Geometry check sheet. Reference: the model listing, model coordinates, mm. A direction names the side the tool comes from. Give positions to 0.01 mm unless a question says otherwise; leave off trailing zeros. Loops run counter-clockwise (first coordinate to the right, second up) from the corner with the lowest first, then second, coordinate; pieces in that order, holes last. Notation, with made-up numbers: (-22, -2.5) - (0, -2.5) arc R27 cw to (0, 35.5) - close; hole circle Ø7 at (83.25, 24). An arc over 180 degrees is marked (long way). Use a Markdown table: item, result. Add a question column.
1. Draft check along X on faces 6 (the cylindrical face through (6.3, 99.98, -32.47)), 7 (the flat face through (-1, 38, -32)), 8 (the flat face through (24.5, 14, -0.4)). Enter one of: pulls with the +X half, pulls with the -X half, needs draft (parallel to the pull), parting line crosses it, or undercut.
2. Cross-section at A-A on z = 0.5. Enter the section's corners in (x, y).
3. Material ranges on L1, parallel to Y at x = 16, z = -9; L2, parallel to Z at x = 11.5, y = 51; L3, parallel to X at y = 79, z = 2.5, recorded low to high.
4. Cross-section at C-C on z = 18. Enter the section's corners in (x, y).
5. Cross-section at B-B on y = 65.5. Enter the section's corners in (x, z).
6. Depth check by flat-ended pin: P1, Ø7.5, axis at x = 28.09, z = -0.34, coming from the +Y side; P2, Ø20, axis at x = 17.5, y = 41.5, coming from the +Z side; P3, Ø12, axis at x = 28.5, z = -1.5, coming from the +Y side. Enter the tip coordinate at first touch or a pass-through.
7. Set-up check for faces 1 (the cylindrical face through (-6.285, 99.993, -32.464)), 2 (the cylindrical face through (19.675, 87.022, -22.273)), 3 (the flat face through (-32, 75, -31)), 4 (the flat face through (32, 74, -31)), 5 (the cylindrical face through (22.726, 17.042, -1.534)): record each of +Z, -Z, +X, -X, +Y, -Y from which the full face is reachable in a straight line by a thin tool's end or side.
8. Cross-section at D-D on x = 41.5. Enter the section's corners in (y, z), and give its area (3 significant figures).
from build123d import *

# Parameters (mm, degrees)
SKETCH4_W                      = 96
SKETCH4_H                      = 64
BOSS_EXTRUDE1_DEPTH            = 20
BOSS_EXTRUDE2_DEPTH            = 32
BOSS_EXTRUDE3_DEPTH            = 12
SKETCH7_R                      = 26
SKETCH7_R_2                    = 16
BOSS_EXTRUDE4_DEPTH            = 32
CUT_EXTRUDE1_START             = -32
SKETCH8_R                      = 16
CUT_EXTRUDE1_DEPTH             = 32
RIB1_START                     = -6
RIB1_DEPTH                     = 12
FILLET1_R                      = 1
CBORE_FOR_M6_SHCS2_D           = 6.6
CBORE_FOR_M6_SHCS2_CBORE_D     = 11
CBORE_FOR_M6_SHCS2_CBORE_DEPTH = 6


with BuildPart() as part:
    # Sketch4 → Boss-Extrude1 (new body)
    with BuildSketch(Plane(origin=(0, 0, 0), x_dir=(1, 0, 0), z_dir=(0, 1, 0))):
        Rectangle(SKETCH4_W, SKETCH4_H)
    extrude(amount=BOSS_EXTRUDE1_DEPTH)

    # Sketch5 → Boss-Extrude2 (add, symmetric)
    with BuildSketch(Plane(origin=(0, 0, 0), x_dir=(0, 0, -1), z_dir=(1, 0, 0))):
        with BuildLine():
            Line((20, 0), (32, 0))
            Line((32, 0), (32, 76.178360588))
            ThreePointArc((32, 76.178360588), (33.228648741, 82.123937475), (36.713317934, 87.095510953))
            Line((36.713317934, 87.095510953), (63.616851895, 112.445358766))
            Line((63.616851895, 112.445358766), (55.387506243, 121.179079058))
            Line((55.387506243, 121.179079058), (28.483972282, 95.829231245))
            ThreePointArc((28.483972282, 95.829231245), (22.211567734, 86.880398983), (20, 76.178360588))
            Line((20, 76.178360588), (20, 0))
        make_face()
    extrude(amount=BOSS_EXTRUDE2_DEPTH, both=True)

    # Sketch6 → Boss-Extrude3 (add)
    with BuildSketch(Plane(origin=(0, 36.544630029, 34.434168053), x_dir=(1, 0, 0), z_dir=(0, 0.7278100243036815, 0.6857788043699474))):
        with BuildLine():
            Line((-32, 123.413626216), (32, 123.413626216))
            ThreePointArc((32, 123.413626216), (0, 155.413626216), (-32, 123.413626216))
        make_face()
    extrude(amount=-BOSS_EXTRUDE3_DEPTH)

    # Sketch7 → Boss-Extrude4 (add)
    with BuildSketch(Plane(origin=(0, 36.544630029, 34.434168053), x_dir=(1, 0, 0), z_dir=(0, 0.7278100243036815, 0.6857788043699474))):
        with Locations(Location((0, 123.413626216, 0), (0, 0, 270))):
            Circle(SKETCH7_R)
        with Locations(Location((0, 123.413626216, 0), (0, 0, 270))):
            Circle(SKETCH7_R_2, mode=Mode.SUBTRACT)
    extrude(amount=BOSS_EXTRUDE4_DEPTH)

    # Sketch8 → Cut-Extrude1 (cut)
    with BuildSketch(Plane(origin=(0, 36.544630029, 34.434168053), x_dir=(1, 0, 0), z_dir=(0, 0.7278100243036815, 0.6857788043699474)).offset(CUT_EXTRUDE1_START)):
        with Locations(Location((0, 123.413626216, 0), (0, 0, 270))):
            Circle(SKETCH8_R)
    extrude(amount=CUT_EXTRUDE1_DEPTH, mode=Mode.SUBTRACT)

    # Rib1: read off the stored shape, not the designer's step
    # Rib1 outline → Rib1 (add)
    with BuildSketch(Plane(origin=(0, 0, 0), x_dir=(0, 0, -1), z_dir=(1, 0, 0)).offset(RIB1_START)):
        with BuildLine():
            Line((28.483972282, 95.829231245), (36.975207197, 103.830095115))
            Line((36.975207197, 103.830095115), (19.144958284, 122.753155747))
            Line((19.144958284, 122.753155747), (10.653723368, 114.752291877))
            ThreePointArc((10.653723368, 114.752291877), (-1.658774448, 97.186065586), (-6, 76.178360588))
            ThreePointArc((-6, 76.178360588), (-12.815134364, 45.226752398), (-32, 20))
            Line((-32, 20), (20, 20))
            Line((20, 20), (20, 76.178360588))
            ThreePointArc((20, 76.178360588), (22.211567734, 86.880398983), (28.483972282, 95.829231245))
        make_face()
    extrude(amount=RIB1_DEPTH)

    # Fillet1
    # the kernel refuses this fillet: 1 mm, written as the material it adds along each edge
    with BuildSketch(Plane(origin=(7, 21, -19), x_dir=(-1, 0, 0), z_dir=(0, 0, -1))) as fillet1_piece_1_section:
        Polygon((0, 0), (FILLET1_R * 1.02, 0), (FILLET1_R * 1.02, -FILLET1_R * 1.02), (0, -FILLET1_R * 1.02), align=None)
    fillet1_piece_1 = extrude(amount=FILLET1_R * 1.02, mode=Mode.PRIVATE)
    fillet1_piece_1 = fillet1_piece_1 - Plane(origin=(7, 21, -19), x_dir=(0.7071067811865475, 0.7071067811865475, 0), z_dir=(0, 0, -1)) * Sphere(FILLET1_R, mode=Mode.PRIVATE)
    add(fillet1_piece_1)
    with BuildSketch(Plane(origin=(-7, 21, -19), x_dir=(1, 0, 0), z_dir=(0, 0, -1))) as fillet1_piece_2_section:
        Polygon((0, 0), (FILLET1_R * 1.02, 0), (FILLET1_R * 1.02, FILLET1_R * 1.02), (0, FILLET1_R * 1.02), align=None)
    fillet1_piece_2 = extrude(amount=FILLET1_R * 1.02, mode=Mode.PRIVATE)
    fillet1_piece_2 = fillet1_piece_2 - Plane(origin=(-7, 21, -19), x_dir=(-0.7071067811865475, 0.7071067811865475, 0), z_dir=(0, 0, -1)) * Sphere(FILLET1_R, mode=Mode.PRIVATE)
    add(fillet1_piece_2)
    with BuildSketch(Plane(origin=(7, 20, -20), x_dir=(0, 0, 1), z_dir=(1, 0, 0)), Plane(origin=(-32, 20, -20), x_dir=(0, 0, 1), z_dir=(1, 0, 0))) as fillet1_piece_3:
        with BuildLine():
            CenterArc((FILLET1_R, -FILLET1_R), FILLET1_R, 90, 90)
            Line((0, -FILLET1_R), (0, 0))
            Line((0, 0), (FILLET1_R, 0))
        make_face()
    extrude(amount=25)
    with BuildSketch(Plane(origin=(0, 121.179079058, -55.387506243), x_dir=(0.13576209912112866, -0.6794294979898851, 0.7210715704445971), z_dir=(-0.990741465995153, -0.09310277001404191, 0.09880901666086746))) as fillet1_piece_4:
        with BuildLine():
            CenterArc((26 + FILLET1_R, FILLET1_R), FILLET1_R, 180, 90)
            Line((26, FILLET1_R), (26, 0))
            Line((26, 0), (26 + FILLET1_R, 0))
        make_face()
    revolve(axis=Axis((0, 121.179079058, -55.387506243), (0, 0.7278100243036815, 0.6857788043699474)), revolution_arc=344.394618628)
    with BuildSketch(Plane(origin=(6, 21, -20), x_dir=(0, 0, 1), z_dir=(0, 1, 0)), Plane(origin=(-6, 21, -20), x_dir=(-1, 0, 0), z_dir=(0, 1, 0))) as fillet1_piece_5:
        with BuildLine():
            CenterArc((FILLET1_R, FILLET1_R), FILLET1_R, 180, 90)
            Line((0, FILLET1_R), (0, 0))
            Line((0, 0), (FILLET1_R, 0))
        make_face()
    extrude(amount=55.178360588)
    with BuildSketch(Plane(origin=(6, 76.178360589, -47.000000001), x_dir=(0, -1.928886679962007e-11, 1.0), z_dir=(0, -1.0, -1.928886679962007e-11))) as fillet1_piece_6:
        with BuildLine():
            CenterArc((27.000000001 + FILLET1_R, -FILLET1_R), FILLET1_R, 90, 90)
            Line((27.000000001, -FILLET1_R), (27.000000001, 0))
            Line((27.000000001, 0), (27.000000001 + FILLET1_R, 0))
        make_face()
    revolve(axis=Axis((6, 76.178360589, -47.000000001), (-1, 0, 0)), revolution_arc=46.703113482)
    with BuildSketch(Plane(origin=(6, 95.829231245, -28.483972282), x_dir=(0, 0.7278100243012071, 0.6857788043725734), z_dir=(0, 0.6857788043725734, -0.7278100243012071)), Plane(origin=(-6, 95.829231245, -28.483972282), x_dir=(-1.0, -2.1788147308559408e-10, -2.0529876082846627e-10), z_dir=(0, 0.6857788043725734, -0.7278100243012071))) as fillet1_piece_7:
        with BuildLine():
            CenterArc((FILLET1_R, FILLET1_R), FILLET1_R, 180, 90)
            Line((-FILLET1_R * 2.99381074515e-10, FILLET1_R), (0, 0))
            Line((0, 0), (FILLET1_R, 0))
        make_face()
    extrude(amount=14.166828749)
    with BuildSketch(Plane(origin=(6, 20, 34.5), x_dir=(1, 0, 0), z_dir=(0, 0, -1))) as fillet1_piece_8_section:
        with BuildLine():
            CenterArc((FILLET1_R, -FILLET1_R), FILLET1_R, 90, 90)
            Line((0, -FILLET1_R), (0, 0))
            Line((0, 0), (FILLET1_R, 0))
        make_face()
    fillet1_piece_8 = extrude(amount=53.5, mode=Mode.PRIVATE)
    fillet1_piece_8 = fillet1_piece_8 - Plane(origin=(6, 76.178360589, 79.692465356), x_dir=(0, -1.8148557691731866e-11, -1.0), z_dir=(-1, 0, 0)) * Cylinder(73.692465356, 111, mode=Mode.PRIVATE)
    add(fillet1_piece_8)
    with BuildSketch(Plane(origin=(-6, 20, 34.5), x_dir=(-1, 0, 0), z_dir=(0, 0, -1))) as fillet1_piece_9_section:
        with BuildLine():
            CenterArc((FILLET1_R, FILLET1_R), FILLET1_R, 180, 90)
            Line((0, FILLET1_R), (0, 0))
            Line((0, 0), (FILLET1_R, 0))
        make_face()
    fillet1_piece_9 = extrude(amount=53.5, mode=Mode.PRIVATE)
    fillet1_piece_9 = fillet1_piece_9 - Plane(origin=(-6, 76.178360589, 79.692465356), x_dir=(0, -1.8148557691731866e-11, -1.0), z_dir=(-1, 0, 0)) * Cylinder(73.692465356, 111, mode=Mode.PRIVATE)
    add(fillet1_piece_9)
    with BuildSketch(Plane(origin=(-6, 76.178360589, -47.000000001), x_dir=(0, -1.928886679962007e-11, 1.0), z_dir=(0, -1.0, -1.928886679962007e-11))) as fillet1_piece_10:
        with BuildLine():
            CenterArc((27.000000001 + FILLET1_R, FILLET1_R), FILLET1_R, 180, 90)
            Line((27.000000001 + FILLET1_R, 0), (27.000000001, 0))
            Line((27.000000001, 0), (27.000000001, FILLET1_R))
        make_face()
    revolve(axis=Axis((-6, 76.178360589, -47.000000001), (-1, 0, 0)), revolution_arc=46.703113482)

    # CBORE for M6 SHCS2 (through all)
    with Locations(Plane(origin=(28.094759236, 20, -0.341970782), x_dir=(0, 0, 1), z_dir=(0, 1, 0))):
        with Locations((0, 0)):
            CounterBoreHole(CBORE_FOR_M6_SHCS2_D / 2, CBORE_FOR_M6_SHCS2_CBORE_D / 2, CBORE_FOR_M6_SHCS2_CBORE_DEPTH)


solid = part.part
Values found:
| question | item | result |
|---|---|---|
| 1 | face 6 | pulls with the +X half |
| 1 | face 7 | needs draft |
| 1 | face 8 | undercut |
| 2 | outline | (-48, 0) - (24.9, 0) - (24.9, 14) - (22.66, 14) - (22.66, 20) - (7, 20) arc R1 cw to (6, 21) - (6, 99.69) - (-6, 99.69) - (-6, 21) arc R1 cw to (-7, 20) - (-48, 20) - close; (31.29, 0) - (48, 0) - (48, 20) - (33.53, 20) - (33.53, 14) - (31.29, 14) - close |
| 3 | L1 | y = 0 to 20 |
| 3 | L2 | z = -32 to -20 |
| 3 | L3 | x = -6 to 6 |
| 4 | outline | (-48, 0) - (48, 0) - (48, 20) - (7, 20) arc R1 cw to (6, 21) - (6, 35.87) - (-6, 35.87) - (-6, 21) arc R1 cw to (-7, 20) - (-48, 20) - close |
| 5 | outline | (-32, -32) - (32, -32) - (32, -20) - (7, -20) arc R1 cw to (6, -19) - (6, 6.78) - (-6, 6.78) - (-6, -19) arc R1 cw to (-7, -20) - (-32, -20) - close |
| 6 | P1 | stops at y = 14 |
| 6 | P2 | stops at z = -20 |
| 6 | P3 | stops at y = 20 |
| 7 | face 1 | +Z, -X |
| 7 | face 2 | +Z, +X |
| 7 | face 3 | +Z, -Z, -X, +Y |
| 7 | face 4 | +Z, -Z, +X, +Y |
| 7 | face 5 | +Y |
| 8 | outline | (0, -32) - (20, -32) - (20, 32) - (0, 32) - close |
| 8 | area | 1,280 mm2 |
